Verification items for the finished model (mm, model axes). Face numbers are marked on the shaded views. A direction names the side the tool comes from. Give positions to 0.01 mm unless a question says otherwise; leave off trailing zeros. Loops run counter-clockwise (first coordinate to the right, second up) from the corner with the lowest first, then second, coordinate; pieces in that order, holes last. Notation, with made-up numbers: (18, -14.75) - (55, -14.75) arc R8 cw to (55, -5.75) - close; hole circle Ø1 at (-22.5, 38). An arc over 180 degrees is marked (long way). Use one line per item in the form item = value.
```python
from build123d import *

# Parameters (mm, degrees)
F1_DEPTH = 25.4


with BuildPart() as f1:
    # F0 (on Front) → F1 (new body)
    with BuildSketch(Plane.XZ):
        with BuildLine():
            add(Edge.make_bspline(
                [(-41.275, 9.525), (-22.0747437676, 40.2046527133), (10.3334958868, 60.2024181647), (44.4254317337, 67.4494675196)],
                knots=[0, 0, 0, 0, 100.1940888091, 100.1940888091, 100.1940888091, 100.1940888091], degree=3))
            Line((-41.275, 9.525), (22.225, 9.525))
            Line((22.225, 9.5250000022), (22.225, 34.925))
            ThreePointArc((22.225, 34.925), (28.3041929243, 54.6144651819), (44.4254317337, 67.4494675196))
        make_face()
        Polygon((22.225, 9.525), (-41.275, 9.525), (-41.275, -9.525), (41.275, -9.525), (41.275, 9.525), align=None)
        with BuildLine():
            Line((22.225, 34.925), (22.225, 9.5250000022))
            Line((22.225, 9.525), (41.275, 9.525))
            Line((41.275, 9.525), (41.275, 34.925))
            ThreePointArc((41.275, 34.925), (45.9246798487, 46.1503201513), (57.15, 50.8))
            Line((57.15, 50.8), (62.4140998637, 50.8))
            Line((62.4140998637, 50.8), (62.4140998637, 59.7440389732))
            Line((62.4140998637, 59.7440389732), (86.6818488397, 59.7440389732))
            Line((86.6818488397, 59.7440389732), (85.8401209116, 69.85))
            Line((85.8401209116, 69.85), (59.9131250273, 69.85))
            add(Edge.make_bspline(
                [(44.4254317337, 67.4494675196), (49.5629070715, 68.5415597229), (54.7386173045, 69.3440971379), (59.9131250273, 69.85)],
                knots=[100.1940888091, 100.1940888091, 100.1940888091, 100.1940888091, 115.2928107637, 115.2928107637, 115.2928107637, 115.2928107637], degree=3))
            ThreePointArc((44.4254317337, 67.4494675196), (28.3041929243, 54.6144651819), (22.225, 34.925))
        make_face()
        with BuildLine():
            ThreePointArc((57.15, 69.85), (50.675488556, 69.2446201401), (44.4254317337, 67.4494675196))
            add(Edge.make_bspline(
                [(44.4254317337, 67.4494675196), (49.5629070715, 68.5415597229), (54.7386173045, 69.3440971379), (59.9131250273, 69.85)],
                knots=[100.1940888091, 100.1940888091, 100.1940888091, 100.1940888091, 115.2928107637, 115.2928107637, 115.2928107637, 115.2928107637], degree=3))
            Line((59.9131250273, 69.85), (57.15, 69.85))
        make_face()
        Polygon((87.4268, 50.8), (86.6818488397, 59.7440389732), (62.4140998637, 59.7440389732), (62.4140998637, 50.8), align=None)
        Polygon((113.2140998637, 59.7440389732), (86.6818488397, 59.7440389732), (87.4268, 50.8), (62.4140998637, 50.8), (62.4140998637, 31.1690389732), (113.2140998637, 31.1690389732), align=None)
    extrude(amount=F1_DEPTH)


solid = f1.part
```
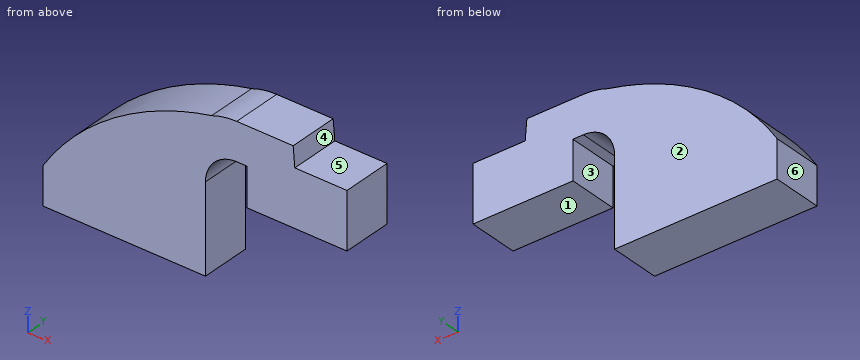
1. Tool access check on the marked faces 1 and 2. Record the directions out of +Z, -Z, +X, -X, +Y, -Y that give a thin tool (end or side, any length) a straight path to the whole face; none if there is none.
Result set:
face_1 = -Z, +X, +Y, -Y
face_2 = +Z, -Z, +X, -X, +Y
2. Scan lines: probe 1 along Z at (x, y) = (102, -17); probe 2 along X at (y, z) = (-7.5, 36); probe 3 along X at (y, z) = (-18, -5) (3 decimals). Record each from-to range of solid material in increasing order.
Result set:
probe_1 = 31.17 to 59.74
probe_2 = -18.74 to 41.31, 62.41 to 113.21
probe_3 = -41.275 to 41.275
3. Section check A-A, the plane z = 8. Record the cut outline in (x, y) (3 decimals).
Result set:
outline = (-41.275, -25.4) - (41.275, -25.4) - (41.275, 0) - (-41.275, 0) - close
4. Draft check along X on the marked faces 3, 4, 5 and 6. Enter one of: released by +X, released by -X, zero draft, split by the parting line, or undercut.
Result set:
face_3 = undercut
face_4 = released by +X
face_5 = zero draft
face_6 = released by -X
5. Section check B-B, the plane x = 80. Record the cut outline in (y, z).
Result set:
outline = (-25.4, 31.17) - (0, 31.17) - (0, 69.85) - (-25.4, 69.85) - close
6. Depth check by flat-ended pin: pin 1 Ø1 at (y, z) = (-18, 27.5) entering from +X (3 decimals); pin 2 Ø1.6 at (x, y) = (60, -18.5) entering from -Z; pin 3 Ø10 at (y, z) = (-18, 42.5) entering from -X. Enter the tip coordinate at first touch or a pass-through.
Result set:
pin_1 = 41.275
pin_2 = 50.8
pin_3 = -17.02
